For this review, take the finished solid that the model builds, in its own axes (mm). A direction names the side the tool comes from. Coordinates: 2 decimals unless noted, no trailing zeros. Order: outer loops, then holes, each group sorted by start corner. A loop starts at its lowest first (then second) coordinate and runs counter-clockwise, first axis right, second up. Notation, with made-up numbers: (84, 33.5) -> (134, 33.5) arc R14 cw to (134, 41.5) -> close; hole circle Ø5 at (17, 47). An arc over 180 degrees is marked (long way). Return JSON: item names as keys, results as strings. Group by question number.
Item 1: For line 1 along Z through (x, y) = (0, 3.75); line 2 along Y through (x, z) = (-6, 7.5), list the stretches that pass through material, from the lowest coordinate up.
Item 2: Take a section at A-A (z = 0). Write out the cut boundary in (x, y), then the cut area to 3 significant figures.
Item 3: Machinability: for faces 1 (the flat face through (7, -6, -3)), 2 (the flat face through (8, 0, 14)), 3 (the flat face through (-9.774, -7.177, 8.339)), 4 (the flat face through (-5, -6, -3)), 5 (the flat face through (7, -6, 10)), which of the approach directions +Z, -Z, +X, -X, +Y, -Y give a long, thin tool a straight path to every point of the face, cutting with its end or side? Answer none if there is none.
Item 4: Draft analysis for pull direction X (two halves, no side actions). For faces 6 (the flat face through (0, -12.5, 9)), 7 (the flat face through (9.726, -7.323, 8.339)), 8 (the flat face through (0, -6, -1)), state which applies: +X half, -X half, draft (parallel to the pull), parting line (faces both ways), or undercut.
Item 5: Insertion check: pin 1 (0.6 mm diameter, centred on x = -21, z = 21, fed in from +Y); pin 2 (2 mm diameter, centred on x = -1.5, y = -4, fed in from -Z); pin 3 (1 mm diameter, centred on y = -1, z = 6.5, fed in from -X). Each pin has a flat end and moves straight along its axis. Give the tip position at first contact, or say it passes through.
Item 6: Take a section at D-D (y = -4). Write out the cut boundary in (x, z), then the cut area to 3 significant figures.
Item 7: Take a section at B-B (x = 0). Write out the cut boundary in (y, z).
Item 8: Take a section at C-C (y = 7.75). Write out the cut boundary in (x, z).
```python
from build123d import *

# Parameters (mm, degrees)
SKETCH1_R             = 2.6
SKETCH1_R_2           = 1.5
BOSS_EXTRUDE1_DEPTH   = 9
BOSS_EXTRUDE1_2_DEPTH = 9
BOSS_EXTRUDE1_3_DEPTH = 9
SKETCH2_W             = 23
SKETCH2_H             = 25
BOSS_EXTRUDE2_DEPTH   = 12.5
CUT_EXTRUDE1_START    = -2
SKETCH3_W             = 14
SKETCH3_H             = 8.5
CUT_EXTRUDE1_DEPTH    = 24
BOSS_EXTRUDE3_START   = 11.5
SKETCH4_W             = 2
SKETCH4_H             = 10.5
BOSS_EXTRUDE3_DEPTH   = 26
BOSS_EXTRUDE4_START   = -11.5
SKETCH4_2_W           = 2
SKETCH4_2_H           = 10.5
BOSS_EXTRUDE4_DEPTH   = 26
SKETCH5_W             = 2
SKETCH5_H             = 12.5
BOSS_EXTRUDE5_DEPTH   = 15
CUT_EXTRUDE2_DEPTH    = 23
CUT_EXTRUDE3_DEPTH    = 2


with BuildPart() as part:
    # Sketch1 → Boss-Extrude1 (new body)
    with BuildSketch(Plane(origin=(0, 0, 0), x_dir=(1, 0, 0), z_dir=(0, 1, 0))):
        with Locations((-8.25, -14.289419162)):
            Circle(SKETCH1_R)
        with Locations((-8.25, -14.289419162)):
            Circle(SKETCH1_R_2, mode=Mode.SUBTRACT)
    extrude(amount=BOSS_EXTRUDE1_DEPTH)



with BuildPart() as body_2:
    # Sketch1 → Boss-Extrude1 2 (new body)
    with BuildSketch(Plane(origin=(0, 0, 0), x_dir=(1, 0, 0), z_dir=(0, 1, 0))):
        Circle(SKETCH1_R)
        Circle(SKETCH1_R_2, mode=Mode.SUBTRACT)
    extrude(amount=BOSS_EXTRUDE1_2_DEPTH)


with BuildPart() as body_3:
    # Sketch1 → Boss-Extrude1 3 (new body)
    with BuildSketch(Plane(origin=(0, 0, 0), x_dir=(1, 0, 0), z_dir=(0, 1, 0))):
        with Locations((8.25, -14.289419162)):
            Circle(SKETCH1_R)
        with Locations((8.25, -14.289419162)):
            Circle(SKETCH1_R_2, mode=Mode.SUBTRACT)
    extrude(amount=BOSS_EXTRUDE1_3_DEPTH)


with BuildPart() as part_1:
    add(part.part)

    add(body_2.part)  # Boss-Extrude2 merges body 2

    add(body_3.part)  # Boss-Extrude2 merges body 3
    # Sketch2 → Boss-Extrude2 (add)
    with BuildSketch(Plane(origin=(0, 0, 0), x_dir=(1, 0, 0), z_dir=(0, 1, 0))):
        with Locations((0, -9.5)):
            Rectangle(SKETCH2_W, SKETCH2_H)
    extrude(amount=-BOSS_EXTRUDE2_DEPTH)

    # Sketch3 → Cut-Extrude1 (cut, through all)
    with BuildSketch(Plane(origin=(0, 0, -3), x_dir=(-1, 0, 0), z_dir=(0, 0, -1)).offset(CUT_EXTRUDE1_START)):
        with Locations((0, -6.25)):
            Rectangle(SKETCH3_W, SKETCH3_H)
    extrude(amount=-CUT_EXTRUDE1_DEPTH, mode=Mode.SUBTRACT)

    # Sketch4 → Boss-Extrude3 (add)
    with BuildSketch(Plane.ZY.offset(BOSS_EXTRUDE3_START)):
        with Locations((21, -7.25)):
            Rectangle(SKETCH4_W, SKETCH4_H)
    extrude(amount=BOSS_EXTRUDE3_DEPTH)

    # Sketch4<2> → Boss-Extrude4 (add)
    with BuildSketch(Plane.ZY.offset(BOSS_EXTRUDE4_START)):
        with Locations((21, -7.25)):
            Rectangle(SKETCH4_2_W, SKETCH4_2_H)
    extrude(amount=-BOSS_EXTRUDE4_DEPTH)

    # Sketch5 → Boss-Extrude5 (add)
    with BuildSketch(Plane(origin=(0, 0, -3), x_dir=(-1, 0, 0), z_dir=(0, 0, -1))):
        with Locations((-2.5, -6.25)):
            Rectangle(SKETCH5_W, SKETCH5_H)
    extrude(amount=BOSS_EXTRUDE5_DEPTH)

    # Sketch6 → Cut-Extrude2 (cut)
    with BuildSketch(Plane.XY.offset(-3)):
        Polygon((-11.5, -2), (-8, -12.5), (-11.5, -12.5), align=None)
        Polygon((11.5, -2), (11.5, -12.5), (8, -12.5), align=None)
    extrude(amount=CUT_EXTRUDE2_DEPTH, mode=Mode.SUBTRACT)

    # Sketch7 → Cut-Extrude3 (cut)
    with BuildSketch(Plane.ZY.offset(-1.5)):
        Polygon((-18, 0), (-18, -6.25), (-3, 0), align=None)
    extrude(amount=-CUT_EXTRUDE3_DEPTH, mode=Mode.SUBTRACT)


solid = part_1.part
```
Findings below:
{
 "1": {"line 1": "z = -2.6 to -1.5, 1.5 to 2.6", "line 2": "y = -12.5 to -10.5, -2 to 0"},
 "2": {"outline": "(-11.5, -2) -> (-8, -12.5) -> (8, -12.5) -> (11.5, -2) -> (11.5, 0) -> (2.6, 0) -> (2.6, 9) -> (1.5, 9) -> (1.5, 0) -> (-1.5, 0) -> (-1.5, 9) -> (-2.6, 9) -> (-2.6, 0) -> (-11.5, 0) -> close; hole (-7, -10.5) -> (7, -10.5) -> (7, -2) -> (-7, -2) -> close", "area": "152 mm2"},
 "3": {"face 1": "-Z, +X, +Y, -Y", "face 2": "+Y", "face 3": "-Z, -X, -Y", "face 4": "-Z, -X, +Y, -Y", "face 5": "+Z"},
 "4": {"face 6": "draft", "face 7": "+X half", "face 8": "undercut"},
 "5": {"pin 1": "stops at y = -2", "pin 2": "stops at z = -3", "pin 3": "stops at x = -11.5"},
 "6": {"outline": "(-37.5, 20) -> (-10.83, 20) -> (-10.83, -3) -> (1.5, -3) -> (1.5, -12.6) -> (3.5, -12.6) -> (3.5, -3) -> (10.83, -3) -> (10.83, 20) -> (37.5, 20) -> (37.5, 22) -> (7, 22) -> (7, -1) -> (-7, -1) -> (-7, 22) -> (-37.5, 22) -> close", "area": "346 mm2"},
 "7": {"outline": "(-12.5, -3) -> (0, -3) -> (0, -2.6) -> (9, -2.6) -> (9, -1.5) -> (0, -1.5) -> (0, 1.5) -> (9, 1.5) -> (9, 2.6) -> (0, 2.6) -> (0, 22) -> (-2, 22) -> (-2, -1) -> (-10.5, -1) -> (-10.5, 22) -> (-12.5, 22) -> close"},
 "8": {"outline": "circle Ø5.2 at (-8.25, 14.29); circle Ø5.2 at (0, 0); circle Ø5.2 at (8.25, 14.29); hole circle Ø3 at (-8.25, 14.29); hole circle Ø3 at (0, 0); hole circle Ø3 at (8.25, 14.29)"}
}
